```python
from build123d import *

# Parameters (mm, degrees)
SKETCH_1_W          = 14
SKETCH_1_H          = 36
EXTRUDE_1_DEPTH     = 3
SKETCH_6_R          = 1.6
CUT_EXTRUDE_3_DEPTH = 10
SKETCH_7_R          = 3
CUT_EXTRUDE_4_DEPTH = 1
SKETCH_9_R          = 4.75
EXTRUDE_2_DEPTH     = 12
SKETCH_10_R         = 2.5
CUT_EXTRUDE_5_DEPTH = 12
SKETCH_11_W         = 10.773254888
SKETCH_11_H         = 9.942175225
CUT_EXTRUDE_7_DEPTH = 12
SKETCH_12_W         = 10.083050504
SKETCH_12_H         = 5.143061972
CUT_EXTRUDE_8_DEPTH = 12


with BuildPart() as part:
    # 草图1 → 凸台-拉伸1 (new body)
    with BuildSketch(Plane(origin=(0, 0, 0), x_dir=(1, 0, 0), z_dir=(0, 1, 0))):
        with Locations((7, -18)):
            Rectangle(SKETCH_1_W, SKETCH_1_H)
    extrude(amount=EXTRUDE_1_DEPTH)

    # 草图6 → 切除-拉伸3 (cut)
    with BuildSketch(Plane(origin=(0, 3, 0), x_dir=(1, 0, 0), z_dir=(0, 1, 0))):
        with Locations(Location((4.5, -6, 0), (0, 0, 270))):
            Circle(SKETCH_6_R)
        with Locations(Location((4.5, -30, 0), (0, 0, 270))):
            Circle(SKETCH_6_R)
    extrude(amount=-CUT_EXTRUDE_3_DEPTH, mode=Mode.SUBTRACT)

    # 草图7 → 切除-拉伸4 (cut)
    with BuildSketch(Plane(origin=(0, 3, 0), x_dir=(1, 0, 0), z_dir=(0, 1, 0))):
        with Locations(Location((4.5, -6, 0), (0, 0, 270))):
            Circle(SKETCH_7_R)
        with Locations(Location((4.5, -30, 0), (0, 0, 270))):
            Circle(SKETCH_7_R)
    extrude(amount=-CUT_EXTRUDE_4_DEPTH, mode=Mode.SUBTRACT)

    # 草图9 → 凸台-拉伸2 (add)
    with BuildSketch(Plane(origin=(0, 0, 12), x_dir=(-1, 0, 0), z_dir=(0, 0, -1))):
        with Locations((-14, 4.75)):
            Circle(SKETCH_9_R)
    extrude(amount=-EXTRUDE_2_DEPTH)

    # 草图10 → 切除-拉伸5 (cut)
    with BuildSketch(Plane(origin=(0, 0, 12), x_dir=(-1, 0, 0), z_dir=(0, 0, -1))):
        with Locations(Location((-14, 4.75, 0), (0, 0, 315.572995999))):
            Circle(SKETCH_10_R)
    extrude(amount=-CUT_EXTRUDE_5_DEPTH, mode=Mode.SUBTRACT)

    # 草图11 → 切除-拉伸7 (cut)
    with BuildSketch(Plane(origin=(0, 0, 0), x_dir=(-1, 0, 0), z_dir=(0, 0, -1))):
        with Locations((-14.469441618, 3.035843785)):
            Rectangle(SKETCH_11_W, SKETCH_11_H)
    extrude(amount=-CUT_EXTRUDE_7_DEPTH, mode=Mode.SUBTRACT)

    # 草图12 → 切除-拉伸8 (cut)
    with BuildSketch(Plane.XY.offset(36)):
        with Locations((14.039079275, 2.038040722)):
            Rectangle(SKETCH_12_W, SKETCH_12_H)
    extrude(amount=-CUT_EXTRUDE_8_DEPTH, mode=Mode.SUBTRACT)


solid = part.part
```
Verification items for the finished model (mm, model axes). A direction names the side the tool comes from. Give positions to 0.01 mm unless a question says otherwise; leave off trailing zeros. Loops run counter-clockwise (first coordinate to the right, second up) from the corner with the lowest first, then second, coordinate; pieces in that order, holes last.
1. Section check C-C, the plane y = 4.75. Enter the section's corners in (x, z).
2. Section check A-A, the plane x = 4.5. Enter the section's corners in (y, z), then the cut area to 3 significant figures.
3. Set-up check for faces 4 (the cylindrical face through (4.6, 2.5, 27)), 5 (the flat face through (12, 3, 12)), 6 (the flat face through (4, 1, 36)), 7 (the flat face through (8.998, 1, 30)): record each of +Z, -Z, +X, -X, +Y, -Y from which the full face is reachable in a straight line by a thin tool's end or side.
4. Thickness scan on line 1 (X direction, y = 1.2, z = 30); line 2 (Y direction, x = 3, z = 7.5); line 3 (Y direction, x = 8.75, z = 27). Record the ranges inside material, lowest first.
5. Go/stop test with flat-tipped pins: pin 1 Ø5 at (x, y) = (16, 4) entering from +Z; pin 2 Ø5 at (x, z) = (5, 21.5) entering from +Y; pin 3 Ø1.5 at (y, z) = (1.5, 31) entering from +X. Record where each tip stops, or that it passes through.
6. Section check D-D, the plane y = 1. Enter the section's corners in (x, z), then the cut area to 3 significant figures.
7. Section check B-B, the plane z = 6. Enter the section's corners in (x, y).
8. Mould release check, pull along X, two halves, no side actions. Record for faces 1 (the flat face through (0, 1, 18)), 2 (the flat face through (9.083, 1, 6)), 3 (the cylindrical face through (4.57, 1.01, 28.4)): released by +X, released by -X, zero draft, split by the parting line, or undercut.
Geometry says:
1. outline: (9.25, 12) - (11.5, 12) - (11.5, 24) - (9.25, 24) - close; (16.5, 12) - (18.75, 12) - (18.75, 24) - (16.5, 24) - close
2. outline: (0, 0) - (3, 0) - (3, 3) - (2, 3) - (2, 4.4) - (0, 4.4) - close; (0, 7.6) - (2, 7.6) - (2, 9) - (3, 9) - (3, 27) - (2, 27) - (2, 28.4) - (0, 28.4) - close; (0, 31.6) - (2, 31.6) - (2, 33) - (3, 33) - (3, 36) - (0, 36) - close
2. area: 83.2 mm2
3. face 4: +Y
3. face 5: -Z, +X, +Y, -Y
3. face 6: +Z, +X, -X, +Y, -Y
3. face 7: +Z, +X, +Y, -Y
4. line 1: x = 0 to 2.9, 6.1 to 9
4. line 2: y = 0 to 2
4. line 3: y = 0 to 3
5. pin 1: stops at z = 24
5. pin 2: stops at y = 3
5. pin 3: stops at x = 9
6. outline: (0, 0) - (9.08, 0) - (9.08, 12) - (16.92, 12) - (16.92, 24) - (9, 24) - (9, 36) - (0, 36) - close; hole circle Ø3.2 at (4.5, 6); hole circle Ø3.2 at (4.5, 30)
6. area: 404 mm2
7. outline: (0, 0) - (2.9, 0) - (2.9, 2) - (1.5, 2) - (1.5, 3) - (0, 3) - close; (6.1, 0) - (9.08, 0) - (9.08, 3) - (7.5, 3) - (7.5, 2) - (6.1, 2) - close
8. face 1: released by -X
8. face 2: released by +X
8. face 3: undercut
